Read the model definition and answer for the solid it produces. Units are mm, in the model's axes. A direction names the side the tool comes from. Coordinates: 2 decimals unless noted, no trailing zeros. Loops run counter-clockwise (first coordinate to the right, second up) from the corner with the lowest first, then second, coordinate; pieces in that order, holes last. Notation, with made-up numbers: (48.25, 57) - (75.25, 57) arc R15 cw to (75.25, 74) - close; hole circle Ø6 at (56, -17). An arc over 180 degrees is marked (long way). Use one line per item in the form item = value.
from build123d import *

# Parameters (mm, degrees)
BASE_DEPTH            = 7.5
MOUNT_START           = -2
MOUNT_DEPTH           = 4
MOUNT_HOLE_DEPTH      = 204.131478566
MOUNT_HOLE_DEPTH_BACK = 204.131478566
SKETCH12_R            = 1.5
SKETCH14_R            = 2
SHAFT_HOLE_DEPTH      = 37.394984425
SKETCH13_W            = 2.5
SKETCH13_H            = 3.5


with BuildPart() as part:
    # Sketch9 → base (new, symmetric)
    with BuildSketch(Plane(origin=(0, 0, 0), x_dir=(1, 0, 0), z_dir=(0, 1, 0))):
        with BuildLine():
            ThreePointArc((-187.113473072, -32.993153757), (-190, 0), (-187.113473072, 32.993153757))
            Line((-187.113473072, 32.993153757), (-196.961550602, 34.729635533))
            ThreePointArc((-196.961550602, 34.729635533), (-200, 0), (-196.961550602, -34.729635533))
            Line((-196.961550602, -34.729635533), (-187.113473072, -32.993153757))
        make_face()
    extrude(amount=BASE_DEPTH, both=True)

    # Sketch11 → mount (cut)
    with BuildSketch(Plane(origin=(0, 0, 0), x_dir=(1, 0, 0), z_dir=(0, 1, 0)).offset(MOUNT_START)):
        with BuildLine():
            Line((-189.73665961, -10), (-199.749843554, -10))
            ThreePointArc((-199.749843554, -10), (-198.7407137, -22.408228804), (-196.961550602, -34.729635533))
            Line((-196.961550602, -34.729635533), (-187.113473072, -32.993153757))
            ThreePointArc((-187.113473072, -32.993153757), (-188.775466906, -21.536552519), (-189.73665961, -10))
        make_face()
        with BuildLine():
            Line((-189.73665961, 10), (-199.749843554, 10))
            ThreePointArc((-199.749843554, 10), (-198.7407137, 22.408228804), (-196.961550602, 34.729635533))
            Line((-196.961550602, 34.729635533), (-187.113473072, 32.993153757))
            ThreePointArc((-187.113473072, 32.993153757), (-188.775466906, 21.536552519), (-189.73665961, 10))
        make_face()
    extrude(amount=MOUNT_DEPTH, mode=Mode.SUBTRACT)

    # Sketch12 → mount hole (cut, two sides: drawn at the far end of the back side and taken through both)
    with BuildSketch(Plane(origin=(0, 0, 0), x_dir=(1, 0, 0), z_dir=(0, 1, 0)).offset(-MOUNT_HOLE_DEPTH_BACK)):
        with Locations(Location((-193.331747968, 25.452607483, 0), (0, 0, 270))):
            Circle(SKETCH12_R)
        with Locations(Location((-194.257966128, 16.995369836, 0), (0, 0, 270))):
            Circle(SKETCH12_R)
        with Locations(Location((-194.257966128, -16.995369836, 0), (0, 0, 270))):
            Circle(SKETCH12_R)
        with Locations(Location((-193.331747968, -25.452607483, 0), (0, 0, 270))):
            Circle(SKETCH12_R)
    extrude(amount=MOUNT_HOLE_DEPTH + MOUNT_HOLE_DEPTH_BACK, mode=Mode.SUBTRACT)

    # Sketch14 → shaft hole (cut, through all)
    with BuildSketch(Plane.ZY.offset(195)):
        Circle(SKETCH14_R)
    extrude(amount=-SHAFT_HOLE_DEPTH, mode=Mode.SUBTRACT)

    # Sketch13 → Cut-Revolve1 (revolve, cut)
    with BuildSketch(Plane(origin=(0, 0, 0), x_dir=(1, 0, 0), z_dir=(0, 1, 0)), mode=Mode.PRIVATE) as cut_revolve1_sk:
        with Locations((-193.75, 1.75)):
            Rectangle(SKETCH13_W, SKETCH13_H)
    revolve(cut_revolve1_sk.sketch.rotate(Axis((0, 0, 0), (-1, 0, 0)), 180), axis=Axis((0, 0, 0), (-1, 0, 0)), mode=Mode.SUBTRACT)


solid = part.part
Item 1: The part is cut by section B-B on y = 0. Give the vertices of the cut face in (x, z), plus the area to 3 significant figures.
Results below:
outline = (-199.75, -10) - (-189.74, -10) arc R190 cw to (-189.99, -2) - (-192.5, -2) - (-192.5, -3.5) - (-195, -3.5) - (-195, 3.5) - (-192.5, 3.5) - (-192.5, 2) - (-189.99, 2) arc R190 cw to (-189.74, 10) - (-199.75, 10) arc R200 ccw to start
area = 173 mm²
Item 2: The part is cut by section D-D on z = -13. Give the vertices of the cut face in (x, y), plus the area to 3 significant figures.
Results below:
outline = (-199.58, -7.5) - (-189.55, -7.5) - (-189.55, -2) - (-199.58, -2) - close; (-199.58, 2) - (-189.55, 2) - (-189.55, 7.5) - (-199.58, 7.5) - close
area = 110 mm²
Item 3: Each of these flat-tipped pins is pushed along its axis until it touches: P1, Ø3, axis at y = 2.5, z = 3.5, coming from the +X side; P2, Ø2.5, axis at x = -193.33, z = -25.45, coming from the +Y side; P3, Ø5.5, axis at y = 0.5, z = -1, coming from the +X side; P4, Ø1.2, axis at x = -193, y = -0.5, coming from the +Z side. Where does it stop, or does it pass through?
Results below:
P1 = -189.93
P2 = through
P3 = -189.96
P4 = 10
Item 4: The part is cut by section A-A on z = 0. Give the vertices of the cut face in (x, y).
Results below:
outline = (-200, -7.5) - (-190, -7.5) - (-190, -2) - (-192.5, -2) - (-192.5, -3.5) - (-195, -3.5) - (-195, 3.5) - (-192.5, 3.5) - (-192.5, 2) - (-190, 2) - (-190, 7.5) - (-200, 7.5) - close
Item 5: For a pull along Z with two mould halves and no side action, classify faces 1 (the flat face through (-194, 2, 22)), 2 (the flat face through (-191.97, 4.79, -33.85)), 3 (the cylindrical face through (-194.796, -4.788, -25.778)) as +Z half, -Z half, draft (parallel to the pull), parting line (faces both ways), or undercut.
Results below:
face_1 = draft
face_2 = -Z half
face_3 = undercut
Item 6: The part is cut by section C-C on x = -188.75. Give the vertices of the cut face in (y, z).
Results below:
outline = (-7.5, -33.28) - (-2, -33.28) - (-2, -21.76) - (-7.5, -21.76) - close; (-7.5, 21.76) - (-2, 21.76) - (-2, 33.28) - (-7.5, 33.28) - close; (2, -33.28) - (7.5, -33.28) - (7.5, -21.76) - (2, -21.76) - close; (2, 21.76) - (7.5, 21.76) - (7.5, 33.28) - (2, 33.28) - close
Item 7: Find the intervals of material crossed by L1, parallel to Y at x = -193, z = -27.5; L2, parallel to Z at x = -195.5, y = -3.75; L3, parallel to Y at x = -194, z = 0, in increasing order.
Results below:
L1 = -7.5 to -2, 2 to 7.5
L2 = -34.47 to -17.84, -16.15 to 16.15, 17.84 to 34.47
L3 = -7.5 to -3.5, 3.5 to 7.5
Item 8: Which of the six approach directions +Z, -Z, +X, -X, +Y, -Y give full straight-line access (tool end or side, diameter ignored) to faces 4 (the flat face through (-195, 0, -10)), 5 (the cylindrical face through (-191, -2, 0)), 6 (the flat face through (-195, 0, 10)), 7 (the cylindrical face through (-192.77, -4.79, 16.8)), 8 (the flat face through (-192.5, -2, -2))?
Results below:
face_4 = -Z, +X, -X
face_5 = +X
face_6 = +Z, +X, -X
face_7 = +Y, -Y
face_8 = none
